Input: part model. Units: mm. Frame: model coordinates. Give positions to 0.01 mm unless a question says otherwise; leave off trailing zeros. Order: outer loops, then holes, each group sorted by start corner. A loop starts at its lowest first (then second) coordinate and runs counter-clockwise, first axis right, second up. Notation, with made-up numbers: (-15.5, -1) -> (-2.5, -1) arc R14 ccw to (-2.5, 24) -> close; hole circle Ø3 at (57.5, 14.25). An arc over 180 degrees is marked (long way). Use a Markdown table: item, result. Add a question column.
from build123d import *

# Parameters (mm, degrees)
SKETCH1_R                                      = 4
SKETCH1_R_2                                    = 3.175
BOSS_EXTRUDE1_DEPTH                            = 3.175
CSK_FOR_6_FLAT_HEAD_MACHINE_SCREW1_D           = 3.7973
CSK_FOR_6_FLAT_HEAD_MACHINE_SCREW1_DEPTH       = 10.973
CSK_FOR_6_FLAT_HEAD_MACHINE_SCREW1_CSINK_D     = 7.0866
CSK_FOR_6_FLAT_HEAD_MACHINE_SCREW1_CSINK_ANGLE = 82
CSK_FOR_6_FLAT_HEAD_MACHINE_SCREW1_TIP         = 1.140824014
FILLET1_R                                      = 4


with BuildPart() as part:
    # Sketch1 → Boss-Extrude1 (new body)
    with BuildSketch(Plane.XY):
        with BuildLine():
            Line((11, 44.330639799), (11, -33.647585352))
            ThreePointArc((11, -33.647585352), (0, -35.4), (-11, -33.647585352))
            Line((-11, -33.647585352), (-11, 44.330639799))
            ThreePointArc((-11, 44.330639799), (0, 45.675), (11, 44.330639799))
        make_face()
        Circle(SKETCH1_R, mode=Mode.SUBTRACT)
        with Locations((0, 39.175)):
            Circle(SKETCH1_R_2, mode=Mode.SUBTRACT)
    extrude(amount=BOSS_EXTRUDE1_DEPTH)

    # CSK for #6 Flat Head Machine Screw1
    with Locations(Plane.XY.offset(3.175)):
        with Locations((-6, 25.298221281), (-6, -25.298221281), (6, 25.298221281), (6, -25.298221281)):
            CounterSinkHole(CSK_FOR_6_FLAT_HEAD_MACHINE_SCREW1_D / 2, CSK_FOR_6_FLAT_HEAD_MACHINE_SCREW1_CSINK_D / 2, depth=CSK_FOR_6_FLAT_HEAD_MACHINE_SCREW1_DEPTH, counter_sink_angle=CSK_FOR_6_FLAT_HEAD_MACHINE_SCREW1_CSINK_ANGLE)
            with Locations((0, 0, -(CSK_FOR_6_FLAT_HEAD_MACHINE_SCREW1_DEPTH + CSK_FOR_6_FLAT_HEAD_MACHINE_SCREW1_TIP / 2))):  # 118° drill point
                Cone(0, CSK_FOR_6_FLAT_HEAD_MACHINE_SCREW1_D / 2, CSK_FOR_6_FLAT_HEAD_MACHINE_SCREW1_TIP, mode=Mode.SUBTRACT)

    # Fillet1
    fillet1_edges = [part.edges().sort_by_distance(p)[0] for p in [
        (11, 44.330639799, 1.5875),
        (-11, 44.330639799, 1.5875),
    ]]
    fillet(fillet1_edges, radius=FILLET1_R)


solid = part.part
Q1. Section query B-B (z = 1.85). Give the number of separate pieces and of enclosed holes in the cut face, plus the area to 3 significant figures.
Q2. Section query A-A (y = 0). Return loops of the section in (x, z) (3 decimals).
Q3. Section query C-C (x = -6). Return loops of the section in (y, z) (3 decimals).
Q4. Ray query, line 1 (Y direction, x = 0, z = 0.7) (3 decimals); line 2 (Y direction, x = -6, z = 0.5); line 3 (X direction, y = -26, z = 0.2). Return the intervals inside material, ascending.
Q5. First-contact query: pin 1 (1 mm diameter, centred on x = 8, z = 1.5, fed in from -Y); pin 2 (3.5 mm diameter, centred on x = 6, y = 25.3, fed in from -Z); pin 3 (6 mm diameter, centred on x = -6, y = 25.3, fed in from +Z). Flat tips, straight axial feed; report the tip coordinate or a pass-through.
Q6. Draft query along Y for faces 1 (the cylindrical face through (-7.8, 25.9, 0.6)), 2 (the cylindrical face through (0.2, -35.4, 1.6)), 3 (the flat face through (-11, 3, 2)), 4 (the cylindrical face through (-10.082, 43.633, 1.61)). Return one class per face: +Y half, -Y half, draft (parallel to the pull), parting line (faces both ways), or undercut.
Solution:
| question | item | result |
|---|---|---|
| 1 | separate pieces | 1 |
| 1 | enclosed holes | 6 |
| 1 | area | 1,600 mm² |
| 2 | outline | (-11, 0) -> (-4, 0) -> (-4, 3.175) -> (-11, 3.175) -> close; (4, 0) -> (11, 0) -> (11, 3.175) -> (4, 3.175) -> close |
| 3 | outline | (-34.888, 0) -> (-27.197, 0) -> (-27.197, 1.283) -> (-28.842, 3.175) -> (-34.888, 3.175) -> close; (-23.4, 0) -> (23.4, 0) -> (23.4, 1.283) -> (21.755, 3.175) -> (-21.755, 3.175) -> (-23.4, 1.283) -> close; (27.197, 0) -> (45.279, 0) -> (45.279, 3.175) -> (28.842, 3.175) -> (27.197, 1.283) -> close |
| 4 | line 1 | y = -35.4 to -4, 4 to 36, 42.35 to 45.675 |
| 4 | line 2 | y = -34.89 to -27.2, -23.4 to 23.4, 27.2 to 45.28 |
| 4 | line 3 | x = -11 to -7.76, -4.24 to 4.24, 7.76 to 11 |
| 5 | pin 1 | stops at y = -34.6 |
| 5 | pin 2 | passes through |
| 5 | pin 3 | stops at z = 2.55 |
| 6 | face 1 | undercut |
| 6 | face 2 | -Y half |
| 6 | face 3 | draft |
| 6 | face 4 | +Y half |
